Here's how the part is built. I have some questions about the finished solid (model axes, mm). Give positions to 0.01 mm unless a question says otherwise; leave off trailing zeros. Write each loop counter-clockwise with the first axis right and the second up, starting at its lowest first coordinate (ties: lowest second). Pieces come first, ordered by that corner, then holes. Notation, with made-up numbers: (6, -38) - (32, -38) arc R28 cw to (32, -18) - close; hole circle Ø1 at (73.5, 3). An arc over 180 degrees is marked (long way). One line per item, written item: value. Start each with the question number.
1) Please list where these lines run through material, in increasing order: L1, parallel to Z at x = -20, y = 2.25; L2, parallel to X at y = 2.2, z = -6; L3, parallel to Z at x = -22, y = 1.15. Write a range as [from, to].
2) Imagine slicing it at A-A on z = 0. Write out the boundary of the cut face in (x, y).
3) Imagine slicing it at D-D on z = -7. Write out the boundary of the cut face in (x, y), plus the area to 3 significant figures.
4) I'm going to push flat-ended pins straight in: P1, Ø2, axis at x = -6, y = 3.5, coming from the +Z side; P2, Ø2, axis at x = -14, y = 1.5, coming from the +Z side; P3, Ø1.5, axis at x = -5.5, y = 2.5, coming from the +Z side. Where does each tip first touch, or does it pass through?
5) Imagine slicing it at C-C on x = 0. Write out the boundary of the cut face in (y, z), plus the area to 3 significant figures.
6) Imagine slicing it at B-B on y = 2.6. Write out the boundary of the cut face in (x, z).
7) We'd pull the mould along Z, two halves only. Please class faces 1 (the flat face through (-17, 2, 5)), 2 (the flat face through (-17, 2, -5)), 3 (the cylindrical face through (1.73, 2.46, 7.81)), 4 (the flat face through (-6, 5, 6)): +Z half, -Z half, draft (parallel to the pull), parting line (faces both ways), or undercut.
Autodesk Inventor part; units mm, degrees
ref_plane "YZ Plane" through (0, 0, 0) normal (1, 0, 0) x (0, 1, 0)
ref_plane "XZ Plane" through (0, 0, 0) normal (0, 1, 0) x (-1, 0, 0)
ref_plane "XY Plane" through (0, 0, 0) normal (0, 0, 1) x (1, 0, 0)
sketch "Sketch1" plane through (0, 0, 0) normal (0, 1, 0) x (-1, 0, 0)
  circle A0 centre (0, 0) radius 8
  line L0 (0, 0) -> (20, 0) construction
  arc A1 (20, -5) -> (20, 5) centre (20, 0) ccw
  line L1 (20, -5) -> (10.9087, -5)
  arc A2 (10.9087, 5) -> (10.9087, -5) centre (0, 0) ccw
  line L2 (20, 5) -> (10.9087, 5)
  circle A3 centre (20, 0) radius 2.3916
  circle A4 centre (0, -2.25) radius 3.175
  point P0 (10.9087, -5)
  point P1 (10.9087, 5)
  dimension "d0" = 16
  dimension "d1" = 20
  dimension "d2" = 24
  dimension "d4" = 10
  dimension "d5" = 6.35
  dimension "d6" = 2.25
extrude "Extrusion1" add sketch "Sketch1" along normal blind 5 contours L1 A2 L2 A1
fillet "Fillet1" radius 6.35 2 edges at (-10.9087, 2.5, -5) (-10.9087, 2.5, 5)
properties part number "Capper Gate Linkage"
Numbers:
1. L1: [-5, -2.39], [2.39, 5]
1. L2: [-11, -5.29], [5.29, 10.39]
1. L3: [-4.58, -1.31], [1.31, 4.58]
2. outline: (-25, 0) - (-22.39, 0) - (-22.39, 5) - (-25, 5) - close; (-17.61, 0) - (-8, 0) - (-8, 5) - (-17.61, 5) - close; (8, 0) - (12, 0) - (12, 5) - (8, 5) - close
3. outline: (-9.79, 0) - (-3.87, 0) - (-3.87, 5) - (-9.79, 5) - close; (3.87, 0) - (9.75, 0) - (9.75, 5) - (3.87, 5) - close
3. area: 59.0 mm^2
4. P1: z = 10.91
4. P2: z = 5.16
4. P3: z = 11.02
5. outline: (0, -12) - (5, -12) - (5, -8) - (0, -8) - close; (0, 8) - (5, 8) - (5, 12) - (0, 12) - close
5. area: 40.0 mm^2
6. outline: (-20, -5) - (-14.42, -5) arc R6.35 cw to (-9.43, -7.42) arc R12 ccw (long way) to (-9.43, 7.42) arc R6.35 cw to (-14.42, 5) - (-20, 5) arc R5 ccw to start; hole circle Ø4.78 at (-20, 0); hole circle Ø16 at (0, 0)
7. face 1: +Z half
7. face 2: -Z half
7. face 3: undercut
7. face 4: draft
